from build123d import *

# Parameters (mm, degrees)
VYSUNOUT1_DEPTH = 7
SKICA5_R        = 5
VYSUNOUT4_DEPTH = 40
ZKOSIT1_SIZE    = 0.7
SKICA3_R        = 5.3
VYSUNOUT2_DEPTH = 1
SKICA4_R        = 5.5
VYSUNOUT3_DEPTH = 21.12


with BuildPart() as part:
    # Skica1 → Vysunout1 (new body)
    with BuildSketch(Plane.XY):
        Polygon((8, -4.618802154), (8, 4.618802154), (0, 9.237604307), (-8, 4.618802154), (-8, -4.618802154), (0, -9.237604307), align=None)
    extrude(amount=VYSUNOUT1_DEPTH)

    # Skica2 → Odebrat otočením1 (revolve, cut)
    with BuildSketch(Plane(origin=(0, 0, 0), x_dir=(1, 0, 0), z_dir=(0, 1, 0))):
        Polygon((8, 0), (20.124355653, 0), (20.124355653, -7), align=None)
    revolve(axis=Axis((0, 0, 0), (0, 0, 1)), mode=Mode.SUBTRACT)

    # Skica5 → Vysunout4 (add)
    with BuildSketch(Plane.XY.offset(7)):
        Circle(SKICA5_R)
    extrude(amount=VYSUNOUT4_DEPTH)

    # Zkosit1
    zkosit1_edges = [part.edges().sort_by_distance(p)[0] for p in [
        (-5, 0, 47),
    ]]
    chamfer(zkosit1_edges, length=ZKOSIT1_SIZE)

    # Skica3 → Vysunout2 (add)
    with BuildSketch(Plane.XY.offset(7)):
        Circle(SKICA3_R)
    extrude(amount=VYSUNOUT2_DEPTH)

    # Skica4 → Vysunout3 (add)
    with BuildSketch(Plane.XY.offset(8)):
        with Locations(Location((0, 0, 0), (0, 0, 180))):
            Circle(SKICA4_R)
    extrude(amount=VYSUNOUT3_DEPTH)

    # Skica6 → Odebrat otočením2 (revolve, cut)
    with BuildSketch(Plane(origin=(0, 0, 0), x_dir=(1, 0, 0), z_dir=(0, 1, 0))):
        Polygon((-5.5, -29.12), (-5.5, -28.253974596), (-5, -29.12), align=None)
    revolve(axis=Axis((0, 0, 29.12), (0, 0, -1)), mode=Mode.SUBTRACT)

    # Skica7 → Otočit kolem osy1 (revolve)
    with BuildSketch(Plane(origin=(0, 0, 0), x_dir=(1, 0, 0), z_dir=(0, 1, 0))):
        with BuildLine():
            ThreePointArc((5.3, -7.4), (5.321093687, -7.195690356), (5.383484861, -7))
            Line((5.383484861, -7), (5.3, -7))
            Line((5.3, -7), (5.3, -7.4))
        make_face()
        with BuildLine():
            ThreePointArc((5.5, -8), (5.351316702, -7.716227766), (5.3, -7.4))
            Line((5.3, -7.4), (5.3, -8))
            Line((5.3, -8), (5.5, -8))
        make_face()
    revolve(axis=Axis((0, 0, 28.253974596), (0, 0, -1)))


solid = part.part
CAD build for the part. Positions are in the model's coordinates, mm. A direction names the side the tool comes from. Round coordinates to 2 decimals unless told otherwise and drop trailing zeros. Write each loop counter-clockwise with the first axis right and the second up, starting at its lowest first coordinate (ties: lowest second). Pieces come first, ordered by that corner, then holes.
(1) Slice it at B-B, the plane z = 42. Write the cut outline in (x, y).
(2) Probe line 1 along Z through (x, y) = (3.5, 5); line 2 along Y through (x, z) = (-0.25, 37.5); line 3 along Y through (x, z) = (-4, 4). List the from-to ranges inside material, lowest first.
(3) Drop flat-ended pins along their axis: P1, Ø5, axis at x = -2, y = 6, coming from the -Z side; P2, Ø3, axis at x = 1, z = 36.5, coming from the +Y side; P3, Ø10, axis at y = -3, z = 33, coming from the +X side; P4, Ø1.5, axis at x = 0.5, y = 6, coming from the +Z side. Give the stop position or say it passes through.
(4) Slice it at A-A, the plane z = 13. Write the cut outline in (x, y).
(5) 3-axis set-ups, long thin cutter, end or side, ignore diameter. For faces 1 (the face through (3.944, -6.961, 3.451)), 2 (the face through (1.19, 5.37, 17.99)): which of +Z, -Z, +X, -X, +Y, -Y reach the whole face in a straight line?
From the geometry:
1. outline: circle Ø10 at (0, 0)
2. line 1: z = 0 to 7
2. line 2: y = -4.99 to 4.99
2. line 3: y = -6.93 to 6.93
3. P1: stops at z = 0
3. P2: stops at y = 5
3. P3: stops at x = 5.32
3. P4: stops at z = 28.65
4. outline: circle Ø11 at (0, 0)
5. face 1: +Z, -Z, +X, -Y
5. face 2: +Z
